Verification items for the finished model (mm, model axes). A direction names the side the tool comes from. Coordinates: 2 decimals unless noted, no trailing zeros. Loops run counter-clockwise (first coordinate to the right, second up) from the corner with the lowest first, then second, coordinate; pieces in that order, holes last. Notation, with made-up numbers: (-12, -4.75) -> (36, -4.75) arc R18 ccw to (36, 26.25) -> close; hole circle Ø4 at (18, 13). An arc over 180 degrees is marked (long way). Answer as a JSON object with one key per item and string values. Group by question number.
Q1. Scan lines: L1, parallel to Z at x = -106.5, y = 28.5; L2, parallel to X at y = 25.75, z = 23; L3, parallel to X at y = 30, z = 63.5. Record each from-to range of solid material in increasing order.
Q2. Release check for a two-part mould opening along X. For faces 3 (the conical face through (-105.37, 24.19, 28.05)), 4 (the cylindrical face through (-101.362, 30.294, 64.165)), 5 (the flat face through (-105.49, 20.96, 62.433)) record: released by +X, released by -X, zero draft, split by the parting line, or undercut.
Q3. Gauge pin test, flat end, axial feed: pin 1 Ø1 at (x, z) = (-104, 20) entering from +Y. Record the tip position at first contact, or that the pin passes through.
Q4. Set-up check for faces 1 (the cylindrical face through (-103.153, 24.676, 34.301)), 2 (the flat face through (-105, 24, 65.933)): record each of +Z, -Z, +X, -X, +Y, -Y from which the full face is reachable in a straight line by a thin tool's end or side.
Q5. Cross-section at B-B on z = 54. Record the boundary of the cut face in (x, y).
Q6. Cross-section at A-A on z = 26. Record the boundary of the cut face in (x, y), and give its area (3 significant figures).
```python
from build123d import *

# Parameters (mm, degrees)
SKETCH2_R                       = 2.35
BOSS_EXTRUDE1_DEPTH             = 55
SKETCH3_R                       = 7.5
BOSS_EXTRUDE2_DEPTH             = 3.5
FILLET1_R                       = 0.5
M3X0_5_TAPPED_HOLE1_D           = 2.5
M3X0_5_TAPPED_HOLE1_DEPTH       = 20
M3X0_5_TAPPED_HOLE1_CSINK_D     = 3.05
M3X0_5_TAPPED_HOLE1_CSINK_ANGLE = 90
M3X0_5_TAPPED_HOLE1_TIP         = 0.751075774


with BuildPart() as part:
    # Sketch2 → Boss-Extrude1 (new body)
    with BuildSketch(Plane.XY.offset(7.432534475)):
        with Locations((-105.393983784, 23.97)):
            Circle(SKETCH2_R)
    extrude(amount=BOSS_EXTRUDE1_DEPTH)

    # Sketch3 → Boss-Extrude2 (add)
    with BuildSketch(Plane.XY.offset(62.432534475)):
        with Locations((-105.393983784, 23.97)):
            Circle(SKETCH3_R)
    extrude(amount=BOSS_EXTRUDE2_DEPTH)

    # Fillet1
    fillet1_edges = [part.edges().sort_by_distance(p)[0] for p in [
        (-107.743983784, 23.97, 62.432534475),
        (-112.893983784, 23.97, 62.432534475),
        (-112.893983784, 23.97, 65.932534475),
    ]]
    fillet(fillet1_edges, radius=FILLET1_R)

    # M3x0.5 Tapped Hole1
    with Locations(Plane(origin=(-105.393983784, 23.97, 7.432534475), x_dir=(-1, 0, 0), z_dir=(0, 0, -1))):
        with Locations((0, 0)):
            CounterSinkHole(M3X0_5_TAPPED_HOLE1_D / 2, M3X0_5_TAPPED_HOLE1_CSINK_D / 2, depth=M3X0_5_TAPPED_HOLE1_DEPTH, counter_sink_angle=M3X0_5_TAPPED_HOLE1_CSINK_ANGLE)
            with Locations((0, 0, -(M3X0_5_TAPPED_HOLE1_DEPTH + M3X0_5_TAPPED_HOLE1_TIP / 2))):  # 118° drill point
                Cone(0, M3X0_5_TAPPED_HOLE1_D / 2, M3X0_5_TAPPED_HOLE1_TIP, mode=Mode.SUBTRACT)


solid = part.part
```
Computed values:
{
 "1": {"L1": "z = 62.43 to 65.93", "L2": "x = -106.93 to -103.86", "L3": "x = -109.85 to -100.93"},
 "2": {"face 3": "undercut", "face 4": "split by the parting line", "face 5": "zero draft"},
 "3": {"pin 1": "stops at y = 26.14"},
 "4": {"face 1": "-Z", "face 2": "+Z, +X, -X, +Y, -Y"},
 "5": {"outline": "circle Ø4.7 at (-105.39, 23.97)"},
 "6": {"outline": "circle Ø4.7 at (-105.39, 23.97); hole circle Ø2.5 at (-105.39, 23.97)", "area": "12.4 mm²"}
}
